Read the model definition and answer for the solid it produces. Units are mm, in the model's axes. Round coordinates to 2 decimals unless told otherwise and drop trailing zeros. Loops run counter-clockwise (first coordinate to the right, second up) from the corner with the lowest first, then second, coordinate; pieces in that order, holes last. Notation, with made-up numbers: (55, 64) -> (61, 64) arc R33 cw to (61, 102) -> close; hole circle Ø4 at (51.5, 32.5). An arc over 180 degrees is marked (long way). Put each result on its own line as item: value.
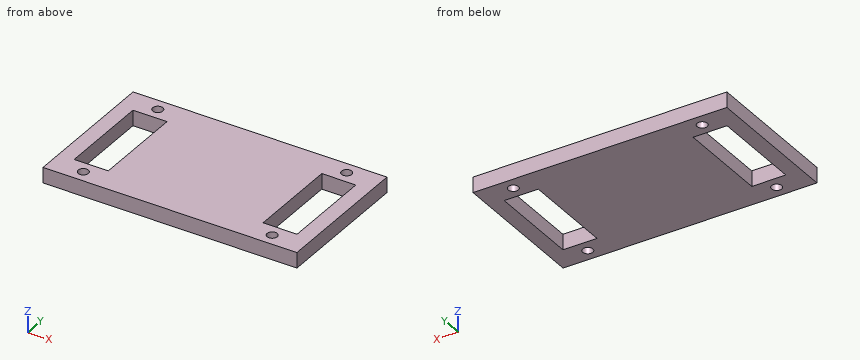
from build123d import *

# Parameters (mm, degrees)
ESQUISSE1_W        = 82
ESQUISSE1_H        = 46
ESQUISSE1_R        = 1.65
ESQUISSE1_W_2      = 11
ESQUISSE1_H_2      = 30
BOSS_EXTRU_1_DEPTH = 5


with BuildPart() as part:
    # Esquisse1 → Boss.-Extru.1 (new body)
    with BuildSketch(Plane.XY):
        with Locations((-41, 59.910969495)):
            Rectangle(ESQUISSE1_W, ESQUISSE1_H)
        with Locations((-10.5, 40.910969495)):
            Circle(ESQUISSE1_R, mode=Mode.SUBTRACT)
        with Locations((-10.5, 78.910969495)):
            Circle(ESQUISSE1_R, mode=Mode.SUBTRACT)
        with Locations((-71.5, 40.910969495)):
            Circle(ESQUISSE1_R, mode=Mode.SUBTRACT)
        with Locations((-71.5, 78.910969495)):
            Circle(ESQUISSE1_R, mode=Mode.SUBTRACT)
        with Locations((-71.5, 59.910969495)):
            Rectangle(ESQUISSE1_W_2, ESQUISSE1_H_2, mode=Mode.SUBTRACT)
        with Locations((-10.5, 59.910969495)):
            Rectangle(ESQUISSE1_W_2, ESQUISSE1_H_2, mode=Mode.SUBTRACT)
    extrude(amount=BOSS_EXTRU_1_DEPTH)


solid = part.part
Item 1: The part is cut by section B-B (z = 2.35). Determine the outline of the cut face in (x, y), then the cut area to 3 significant figures.
Derived:
outline: (-82, 36.91) -> (0, 36.91) -> (0, 82.91) -> (-82, 82.91) -> close; hole (-77, 44.91) -> (-66, 44.91) -> (-66, 74.91) -> (-77, 74.91) -> close; hole circle Ø3.3 at (-71.5, 40.91); hole circle Ø3.3 at (-71.5, 78.91); hole (-16, 44.91) -> (-5, 44.91) -> (-5, 74.91) -> (-16, 74.91) -> close; hole circle Ø3.3 at (-10.5, 40.91); hole circle Ø3.3 at (-10.5, 78.91)
area: 3,080 mm^2
Item 2: Find the intervals of material crossed by line 1 along Y through (x, z) = (-10.5, 1.75); line 2 along X through (y, z) = (45, 3.65); line 3 along Y through (x, z) = (-15, 2.65), in increasing order.
Derived:
line 1: y = 36.91 to 39.26, 42.56 to 44.91, 74.91 to 77.26, 80.56 to 82.91
line 2: x = -82 to -77, -66 to -16, -5 to 0
line 3: y = 36.91 to 44.91, 74.91 to 82.91
Item 3: The part is cut by section A-A (x = -10.5). Determine the outline of the cut face in (y, z), then the cut area to 3 significant figures.
Derived:
outline: (36.91, 0) -> (39.26, 0) -> (39.26, 5) -> (36.91, 5) -> close; (42.56, 0) -> (44.91, 0) -> (44.91, 5) -> (42.56, 5) -> close; (74.91, 0) -> (77.26, 0) -> (77.26, 5) -> (74.91, 5) -> close; (80.56, 0) -> (82.91, 0) -> (82.91, 5) -> (80.56, 5) -> close
area: 47.0 mm^2
Item 4: A flat-ended cylindrical pin translates along its axis: pin 1 Ø2 at (x, y) = (-10.5, 78.91) entering from +Z. Find the tip coordinate at first contact, or state that the pin passes through.
Derived:
pin 1: passes through
